```python
from build123d import *

# Parameters (mm, degrees)
BOSS_EXTRUDE1_DEPTH = 65
CHAMFER2_SIZE       = 10
SKETCH2_R           = 15
CUT_EXTRUDE1_DEPTH  = 5
SKETCH3_R           = 1.5
CUT_EXTRUDE2_DEPTH  = 7.5
FILLET1_R           = 1
SKETCH4_W           = 20
SKETCH4_H           = 40
CUT_EXTRUDE3_DEPTH  = 176.431286259
CUT_EXTRUDE5_REACH  = 200.888
SKETCH5_R           = 1.5
SKETCH5_W           = 27
SKETCH5_H           = 15


with BuildPart() as part:
    # Sketch1 → Boss-Extrude1 (new body)
    with BuildSketch(Plane.XY):
        with BuildLine():
            Line((-40, 137.5), (40, 137.5))
            Line((40, 137.5), (44.969918815, 1.645114527))
            ThreePointArc((44.969918815, 1.645114527), (0, -45), (-44.969918815, 1.645114527))
            Line((-44.969918815, 1.645114527), (-40, 137.5))
        make_face()
    extrude(amount=BOSS_EXTRUDE1_DEPTH)

    # Chamfer2
    chamfer2_edges = [part.edges().sort_by_distance(p)[0] for p in [
        (-42.484959407, 69.572557263, 65),
        (0, -45, 65),
        (-42.484959407, 69.572557263, 0),
        (42.484959407, 69.572557263, 0),
        (0, -45, 0),
        (42.484959407, 69.572557263, 65),
    ]]
    chamfer(chamfer2_edges, length=CHAMFER2_SIZE)

    # Sketch2 → Cut-Extrude1 (cut)
    with BuildSketch(Plane.XY.offset(65)):
        Circle(SKETCH2_R)
    extrude(amount=-CUT_EXTRUDE1_DEPTH, mode=Mode.SUBTRACT)

    # Sketch3 → Cut-Extrude2 (cut)
    with BuildSketch(Plane.XY.offset(60)):
        with Locations((0, 7.5)):
            Circle(SKETCH3_R)
        with Locations((7.5, 0)):
            Circle(SKETCH3_R)
        with Locations((0, -7.5)):
            Circle(SKETCH3_R)
        with Locations((-7.5, 0)):
            Circle(SKETCH3_R)
    extrude(amount=-CUT_EXTRUDE2_DEPTH, mode=Mode.SUBTRACT)

    # Fillet1
    fillet1_edges = [part.edges().sort_by_distance(p)[0] for p in [
        (-15, 0, 60),
        (-15, 0, 65),
    ]]
    fillet(fillet1_edges, radius=FILLET1_R)

    # Sketch4 → Cut-Extrude3 (cut, through all)
    with BuildSketch(Plane(origin=(44.969918815, 1.645114527, 0), x_dir=(0, 0, -1), z_dir=(0.9993315292139455, 0.03655810059230684, 0))):
        with Locations((-32.5, 103.445761243)):
            Rectangle(SKETCH4_W, SKETCH4_H)
    extrude(amount=-CUT_EXTRUDE3_DEPTH, mode=Mode.SUBTRACT)

    # Cut-Extrude5: up to this plane
    cut_extrude5_end = Plane(origin=(-51.096815111, 121.65908428, 42.5), z_dir=(-0.036558100592306846, 0.9993315292139455, 0))
    # Sketch5 → Cut-Extrude5 (cut, up to the surface)
    with BuildSketch(Plane(origin=(0, 137.5, 0), x_dir=(1, 0, 0), z_dir=(0, 1, 0)), mode=Mode.PRIVATE) as cut_extrude5_sk1:
        with Locations(Location((-16.75, -29.25, 0), (0, 0, 270))):
            Circle(SKETCH5_R)
    cut_extrude5_tool1 = split(extrude(cut_extrude5_sk1.sketch, amount=-CUT_EXTRUDE5_REACH, mode=Mode.PRIVATE), bisect_by=cut_extrude5_end, keep=Keep.BOTH, mode=Mode.PRIVATE)
    add(cut_extrude5_tool1.solids().sort_by_distance((-16.75, 137.5, 29.25))[0], mode=Mode.SUBTRACT)
    # Sketch5 → Cut-Extrude5 (cut, up to the surface)
    with BuildSketch(Plane(origin=(0, 137.5, 0), x_dir=(1, 0, 0), z_dir=(0, 1, 0)), mode=Mode.PRIVATE) as cut_extrude5_sk2:
        with Locations((-16.75, -35.75)):
            Circle(SKETCH5_R)
    cut_extrude5_tool2 = split(extrude(cut_extrude5_sk2.sketch, amount=-CUT_EXTRUDE5_REACH, mode=Mode.PRIVATE), bisect_by=cut_extrude5_end, keep=Keep.BOTH, mode=Mode.PRIVATE)
    add(cut_extrude5_tool2.solids().sort_by_distance((-16.75, 137.5, 35.75))[0], mode=Mode.SUBTRACT)
    # Sketch5 → Cut-Extrude5 (cut, up to the surface)
    with BuildSketch(Plane(origin=(0, 137.5, 0), x_dir=(1, 0, 0), z_dir=(0, 1, 0)), mode=Mode.PRIVATE) as cut_extrude5_sk3:
        with Locations(Location((16.75, -35.75, 0), (0, 0, 270))):
            Circle(SKETCH5_R)
    cut_extrude5_tool3 = split(extrude(cut_extrude5_sk3.sketch, amount=-CUT_EXTRUDE5_REACH, mode=Mode.PRIVATE), bisect_by=cut_extrude5_end, keep=Keep.BOTH, mode=Mode.PRIVATE)
    add(cut_extrude5_tool3.solids().sort_by_distance((16.75, 137.5, 35.75))[0], mode=Mode.SUBTRACT)
    # Sketch5 → Cut-Extrude5 (cut, up to the surface)
    with BuildSketch(Plane(origin=(0, 137.5, 0), x_dir=(1, 0, 0), z_dir=(0, 1, 0)), mode=Mode.PRIVATE) as cut_extrude5_sk4:
        with Locations((16.75, -29.25)):
            Circle(SKETCH5_R)
    cut_extrude5_tool4 = split(extrude(cut_extrude5_sk4.sketch, amount=-CUT_EXTRUDE5_REACH, mode=Mode.PRIVATE), bisect_by=cut_extrude5_end, keep=Keep.BOTH, mode=Mode.PRIVATE)
    add(cut_extrude5_tool4.solids().sort_by_distance((16.75, 137.5, 29.25))[0], mode=Mode.SUBTRACT)
    # Sketch5 → Cut-Extrude5 (cut, up to the surface)
    with BuildSketch(Plane(origin=(0, 137.5, 0), x_dir=(1, 0, 0), z_dir=(0, 1, 0)), mode=Mode.PRIVATE) as cut_extrude5_sk5:
        with Locations((0, -32.5)):
            Rectangle(SKETCH5_W, SKETCH5_H)
    cut_extrude5_tool5 = split(extrude(cut_extrude5_sk5.sketch, amount=-CUT_EXTRUDE5_REACH, mode=Mode.PRIVATE), bisect_by=cut_extrude5_end, keep=Keep.BOTH, mode=Mode.PRIVATE)
    add(cut_extrude5_tool5.solids().sort_by_distance((0, 137.5, 32.5))[0], mode=Mode.SUBTRACT)


solid = part.part
```
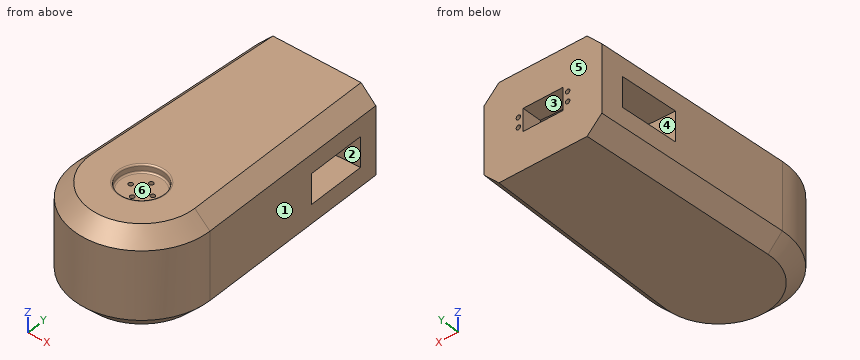
Part model, mm, in its own coordinate system. Face numbers are marked on the shaded views. A direction names the side the tool comes from. Round coordinates to 2 decimals unless told otherwise and drop trailing zeros. Loops run counter-clockwise (first coordinate to the right, second up) from the corner with the lowest first, then second, coordinate; pieces in that order, holes last.
Item 1: Drop flat-ended pins along their axis: P1, Ø1, axis at y = -20, z = 47.5, coming from the -X side; P2, Ø14, axis at x = -4, y = -4, coming from the +Z side; P3, Ø1, axis at x = 2, z = 17.5, coming from the -Y side (3 decimals). Give the stop position or say it passes through.
Item 2: Mould opens along Y. For the marked faces 1, 2 and 3 say: +Y half, -Y half, draft (parallel to the pull), parting line (faces both ways), or undercut.
Item 3: Cut at D-D, the plane y = 72.5. Give the cut face in (x, z), then the cut area to 3 significant figures.
Item 4: Cut at B-B, the plane z = 57. Give the cut face in (x, y).
Item 5: Cut at A-A, the plane y = 19.5. Give the cut face in (x, z), then the cut area to 3 significant figures.
Item 6: 3-axis set-ups, long thin cutter, end or side, ignore diameter. For the marked faces 4, 5 and 6: which of +Z, -Z, +X, -X, +Y, -Y reach the whole face in a straight line?
Item 7: Cut at C-C, the plane z = 19.5. Give the cut face in (x, y).
Item 8: Drill centre lines: line 1 (Z direction, x = -16.75, y = 132.75); line 2 (Z direction, x = -11, y = 122.5); line 3 (X direction, y = 126.75, z = 35.75). Where is each one in solid material? Low to high.
A:
1. P1: stops at x = -40.56
1. P2: stops at z = 60
1. P3: stops at y = -44.975
2. face 1: +Y half
2. face 2: undercut
2. face 3: draft
3. outline: (-42.38, 10) - (-32.37, 0) - (32.37, 0) - (42.38, 10) - (42.38, 55) - (32.37, 65) - (-32.37, 65) - (-42.38, 55) - close
3. area: 5,310 mm2
4. outline: (-42.97, 1.57) arc R43 ccw (long way) to (42.97, 1.57) - (38, 137.5) - (-38, 137.5) - close; hole circle Ø3 at (-7.5, 0); hole circle Ø3 at (0, -7.5); hole circle Ø3 at (0, 7.5); hole circle Ø3 at (7.5, 0)
5. outline: (-44.32, 10) - (-34.31, 0) - (34.31, 0) - (44.32, 10) - (44.32, 55) - (34.31, 65) - (-34.31, 65) - (-44.32, 55) - close
5. area: 5,560 mm2
6. face 4: -X
6. face 5: +Z, -Z, +X, -X, +Y
6. face 6: +Z
7. outline: (-44.97, 1.65) arc R45 ccw (long way) to (44.97, 1.65) - (40, 137.5) - (-40, 137.5) - close
8. line 1: z = 0 to 27.75, 30.75 to 34.25, 37.25 to 65
8. line 2: z = 0 to 22.5, 42.5 to 65
8. line 3: x = -40.39 to -18.25, -15.25 to -13.5, 13.5 to 15.25, 18.25 to 40.39
